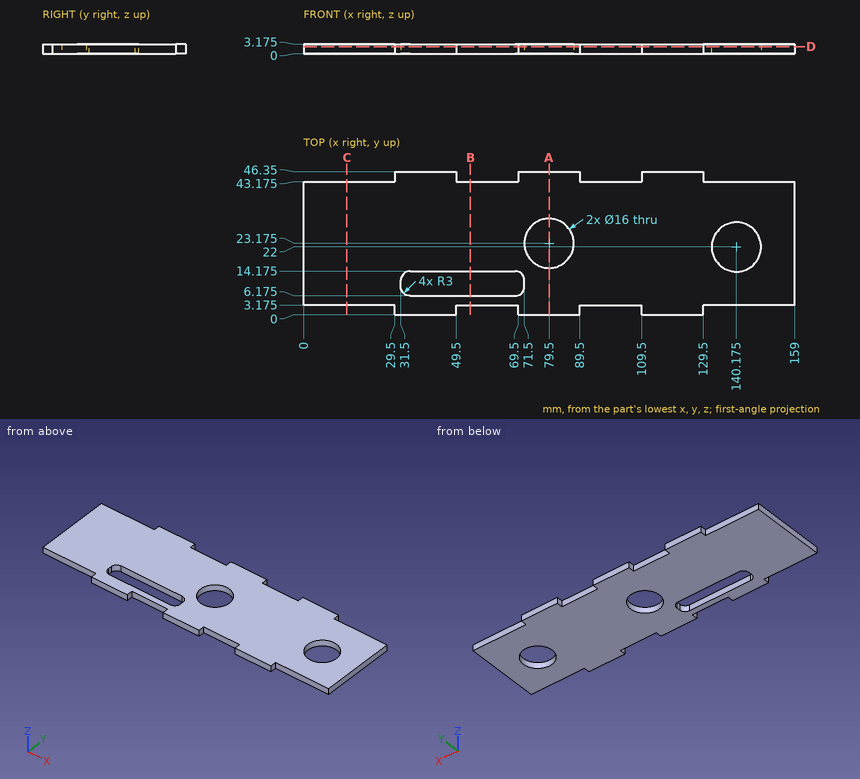
Here's the drawing with two shaded views (mm, measured from the low corner). I have some questions. Coordinates: 2 decimals unless noted, no trailing zeros. Write each loop counter-clockwise with the first axis right and the second up, starting at its lowest first coordinate (ties: lowest second). Pieces come first, ordered by that corner, then holes. Notation, with made-up numbers: M 45,63 L 61,63 A20 cw 61,88 Z; hole C -25.75,19 d3. An arc over 180 degrees is marked long. Answer as CSV lines item,"result".
Item 1: I'm going to push flat-ended pins straight in: P1, Ø1, axis at y = 45, z = 1, coming from the +X side; P2, Ø1, axis at x = 60.5, z = 2, coming from the +Y side (3 decimals); P3, Ø6, axis at x = 56.5, y = 38, coming from the -Z side; P4, Ø1.6, axis at x = 149.5, z = 1.5, coming from the -Y side (3 decimals). Where does each tip first touch, or does it pass through?
Geometry results:
P1,"stops at x = 129.5"
P2,"stops at y = 43.175"
P3,"stops at z = 0"
P4,"stops at y = 3.175"
Item 2: Imagine slicing it at B-B on x = 54. List the corners of the cut face in (y, z) for me (3 decimals).
Geometry results:
outline,"M 3.175,0 L 6.175,0 L 6.175,3.175 L 3.175,3.175 Z; M 14.175,0 L 43.175,0 L 43.175,3.175 L 14.175,3.175 Z"
Item 3: Imagine slicing it at C-C on x = 14. List the corners of the cut face in (y, z) for me (3 decimals), plus the area to 3 significant figures.
Geometry results:
outline,"M 3.175,0 L 43.175,0 L 43.175,3.175 L 3.175,3.175 Z"
area,"127 mm2"
Item 4: Imagine slicing it at A-A on x = 79.5. List the corners of the cut face in (y, z) for me (3 decimals).
Geometry results:
outline,"M 0,0 L 15.175,0 L 15.175,3.175 L 0,3.175 Z; M 31.175,0 L 46.35,0 L 46.35,3.175 L 31.175,3.175 Z"
Item 5: Imagine slicing it at D-D on z = 2.3. State how many separate pieces and enclosed holes the cut face has, plus the area to 3 significant figures.
Geometry results:
separate pieces,"1"
enclosed holes,"3"
area,"6,030 mm2"
Item 6: Please list where these lines run through material, in increasing order: line 1 along X through (y, z) = (43.5, 0.7); line 2 along Y through (x, z) = (79.5, 1) (3 decimals); line 3 along X through (y, z) = (18, 0.3).
Geometry results:
line 1,"x = 29.5 to 49.5, 69.5 to 89.5, 109.5 to 129.5"
line 2,"y = 0 to 15.175, 31.175 to 46.35"
line 3,"x = 0 to 73.4, 85.6 to 133.25, 147.1 to 159"
